from build123d import *

# Parameters (mm, degrees)
EXTRUDE_1_DEPTH = 3
EXTRUDE_START   = 3
SKETCH_2_R      = 1.35
SKETCH_2_R_2    = 3.25
EXTRUDE_2_DEPTH = 4
FILLET_1_R      = 5


with BuildPart() as part:
    # 草圖1 → 填料-伸長1 (new body)
    with BuildSketch(Plane.XY):
        with BuildLine():
            Line((25.7, -30), (25.7, 30))
            ThreePointArc((25.7, 30), (24.030508653, 34.030508653), (20, 35.7))
            Line((20, 35.7), (-20, 35.7))
            ThreePointArc((-20, 35.7), (-24.030508653, 34.030508653), (-25.7, 30))
            Line((-25.7, 30), (-25.7, -30))
            ThreePointArc((-25.7, -30), (-24.030508653, -34.030508653), (-20, -35.7))
            Line((-20, -35.7), (20, -35.7))
            ThreePointArc((20, -35.7), (24.030508653, -34.030508653), (25.7, -30))
        make_face()
    extrude(amount=EXTRUDE_1_DEPTH)

    # 草圖2 → 填料-伸長2 (add)
    with BuildSketch(Plane.XY.offset(EXTRUDE_START)):
        with BuildLine():
            Line((30, -30), (30, 30))
            ThreePointArc((30, 30), (27.071067812, 37.071067812), (20, 40))
            Line((20, 40), (-20, 40))
            ThreePointArc((-20, 40), (-27.071067812, 37.071067812), (-30, 30))
            Line((-30, 30), (-30, -30))
            ThreePointArc((-30, -30), (-27.071067812, -37.071067812), (-20, -40))
            Line((-20, -40), (20, -40))
            ThreePointArc((20, -40), (27.071067812, -37.071067812), (30, -30))
        make_face()
        with Locations((0, 38)):
            Circle(SKETCH_2_R, mode=Mode.SUBTRACT)
        with Locations((0, -38)):
            Circle(SKETCH_2_R, mode=Mode.SUBTRACT)
        Circle(SKETCH_2_R_2, mode=Mode.SUBTRACT)
        with Locations((14, 14)):
            Circle(SKETCH_2_R_2, mode=Mode.SUBTRACT)
    extrude(amount=EXTRUDE_2_DEPTH)

    # 圓角1
    # the kernel refuses this fillet: 5 mm, written as the material it takes off along each edge
    with BuildSketch(Plane(origin=(20, -30, 7), x_dir=(0, -1, 0), z_dir=(-1, 0, 0))) as fillet_1_piece_1:
        with BuildLine():
            CenterArc((5.101020514, -5), FILLET_1_R, 11.536959033, 78.463040967)
            Line((5.101020514, 0), (5.101020514, 0.1))
            Line((5.101020514, 0.1), (10, 0.1))
            Line((10, 0.1), (10.1, 0))
            ThreePointArc((10.1, 0), (10.1, -2), (10.09797959, -3.98))
            Line((10.09797959, -3.98), (10, -4))
        make_face()
    revolve(axis=Axis((20, -30, 7), (0, 0, 1)), revolution_arc=90, mode=Mode.SUBTRACT)
    with BuildSketch(Plane(origin=(30, -30, 7), x_dir=(-1.5640821970914211e-12, 0, -1.0), z_dir=(0, 1, 0)), Plane(origin=(-30, 30, 7), x_dir=(1.5640821970914211e-12, 0, -1.0), z_dir=(0, -1, 0))) as fillet_1_piece_2:
        with BuildLine():
            CenterArc((5, 4.898979486), FILLET_1_R, 180, 78.463040967)
            Line((0, 4.898979486), (-0.1, 4.898979486))
            Line((-0.1, 4.898979486), (-0.1, 0))
            Line((-0.1, 0), (0, -0.1))
            ThreePointArc((0, -0.1), (2, -0.1), (3.98, -0.09797959))
            Line((3.98, -0.09797959), (4, 0))
        make_face()
    extrude(amount=60, mode=Mode.SUBTRACT)
    with BuildSketch(Plane(origin=(20, 30, 7), x_dir=(1, 0, 0), z_dir=(0, -1, 0))) as fillet_1_piece_3:
        with BuildLine():
            CenterArc((5.101020514, -5), FILLET_1_R, 11.536959033, 78.463040967)
            Line((5.101020514, 0), (5.101020514, 0.1))
            Line((5.101020514, 0.1), (10, 0.1))
            Line((10, 0.1), (10.1, 0))
            ThreePointArc((10.1, 0), (10.1, -2), (10.09797959, -3.98))
            Line((10.09797959, -3.98), (10, -4))
        make_face()
    revolve(axis=Axis((20, 30, 7), (0, 0, 1)), revolution_arc=90, mode=Mode.SUBTRACT)
    with BuildSketch(Plane(origin=(20, 40, 7), x_dir=(0, -1.5667467323505197e-12, -1.0), z_dir=(-1, 0, 0)), Plane(origin=(-20, -40, 7), x_dir=(0, 1.5667467323505197e-12, -1.0), z_dir=(1, 0, 0))) as fillet_1_piece_4:
        with BuildLine():
            CenterArc((5, 4.898979486), FILLET_1_R, 180, 78.463040967)
            Line((0, 4.898979486), (-0.1, 4.898979486))
            Line((-0.1, 4.898979486), (-0.1, 0))
            Line((-0.1, 0), (0, -0.1))
            ThreePointArc((0, -0.1), (2, -0.1), (3.98, -0.09797959))
            Line((3.98, -0.09797959), (4, 0))
        make_face()
    extrude(amount=40, mode=Mode.SUBTRACT)
    with BuildSketch(Plane(origin=(-20, 30, 7), x_dir=(0, 1, 0), z_dir=(1, 0, 0))) as fillet_1_piece_5:
        with BuildLine():
            CenterArc((5.101020514, -5), FILLET_1_R, 11.536959033, 78.463040967)
            Line((5.101020514, 0), (5.101020514, 0.1))
            Line((5.101020514, 0.1), (10, 0.1))
            Line((10, 0.1), (10.1, 0))
            ThreePointArc((10.1, 0), (10.1, -2), (10.09797959, -3.98))
            Line((10.09797959, -3.98), (10, -4))
        make_face()
    revolve(axis=Axis((-20, 30, 7), (0, 0, 1)), revolution_arc=90, mode=Mode.SUBTRACT)
    with BuildSketch(Plane(origin=(-20, -30, 7), x_dir=(-1, 0, 0), z_dir=(0, 1, 0))) as fillet_1_piece_6:
        with BuildLine():
            CenterArc((5.101020514, -5), FILLET_1_R, 11.536959033, 78.463040967)
            Line((5.101020514, 0), (5.101020514, 0.1))
            Line((5.101020514, 0.1), (10, 0.1))
            Line((10, 0.1), (10.1, 0))
            ThreePointArc((10.1, 0), (10.1, -2), (10.09797959, -3.98))
            Line((10.09797959, -3.98), (10, -4))
        make_face()
    revolve(axis=Axis((-20, -30, 7), (0, 0, 1)), revolution_arc=90, mode=Mode.SUBTRACT)


solid = part.part
CAD build for the part. Positions are in the model's coordinates, mm. A direction names the side the tool comes from. Round coordinates to 2 decimals unless told otherwise and drop trailing zeros. Order: outer loops, then holes, each group sorted by start corner. A loop starts at its lowest first (then second) coordinate and runs counter-clockwise, first axis right, second up. Notation, with made-up numbers: M -31.75,14 L -3.75,14 A29 ccw -3.75,46 Z; hole C 20.5,5 d7. An arc over 180 degrees is marked long. Use one line per item in the form item = value.
Q1. Probe L1, parallel to Y at x = 0, z = 6; L2, parallel to Y at x = 0, z = 4.25; L3, parallel to Y at x = 17.5, z = 1.75. List the from-to ranges inside material, lowest first.
Recorded:
L1 = -36.65 to -3.25, 3.25 to 36.65
L2 = -39.57 to -39.35, -36.65 to -3.25, 3.25 to 36.65, 39.35 to 39.57
L3 = -35.7 to 35.7
Q2. Saw through at D-D on y = 22.5. Give the cut face in (x, z), then the cut area to 3 significant figures.
Recorded:
outline = M -30,3 L -25.7,3 L -25.7,0 L 25.7,0 L 25.7,3 L 30,3 A5 ccw 25.1,7 L -25.1,7 A5 ccw Z
area = 384 mm^2
Q3. Which spindle directions (+Z, -Z, +X, -X, +Y, -Y) get a long thin tool onto all of the face, cutting with end or side? Do faces 1 (the flat face through (-27, 6, 3)), 2 (the flat face through (-25.7, 0, 1)), 3 (the cylindrical face through (24.07, 33.99, 1.48)). Say none if no direction does.
Recorded:
face_1 = -Z
face_2 = -Z, -X, +Y, -Y
face_3 = -Z, +X, +Y
Q4. Two-plate mould, pull along X, no slides. Class faces 4 (the cylindrical face through (23.99, -34.07, 1.48)), 5 (the cylindrical face through (10.753, 14.143, 4.972)), 6 (the flat face through (-6, 0, 7)): +X half, -X half, draft (parallel to the pull), parting line (faces both ways), or undercut.
Recorded:
face_4 = +X half
face_5 = undercut
face_6 = draft
Q5. Saw through at A-A on y = 14. Give the cut face in (x, z), then the cut area to 3 significant figures.
Recorded:
outline = M -30,3 L -25.7,3 L -25.7,0 L 25.7,0 L 25.7,3 L 30,3 A5 ccw 25.1,7 L 17.25,7 L 17.25,3 L 10.75,3 L 10.75,7 L -25.1,7 A5 ccw Z
area = 358 mm^2
Q6. Saw through at B-B on x = 0. Give the cut face in (y, z), then the cut area to 3 significant figures.
Recorded:
outline = M -40,3 L -39.35,3 L -39.35,4.64 A5 ccw Z; M -36.65,3 L -35.7,3 L -35.7,0 L 35.7,0 L 35.7,3 L 36.65,3 L 36.65,6.75 A5 ccw 35.1,7 L 3.25,7 L 3.25,3 L -3.25,3 L -3.25,7 L -35.1,7 A5 ccw -36.65,6.75 Z; M 39.35,3 L 40,3 A5 ccw 39.35,4.64 Z
area = 482 mm^2
Q7. Flat gauge pins, fed straight in: P1, Ø2.5, axis at y = -7, z = 1.5, coming from the -X side; P2, Ø6, axis at x = 0, y = 0, coming from the -Z side; P3, Ø3, axis at x = 0, y = -38, coming from the +Z side; P4, Ø1, axis at y = -3.5, z = 4, coming from the +X side. Where does each tip first touch, or does it go through?
Recorded:
P1 = -25.7
P2 = 0
P3 = 6.8
P4 = 29.87
Q8. Saw through at C-C on z = 2. Give the cut face in (x, y), then the cut area to 3 significant figures.
Recorded:
outline = M -25.7,-30 A5.7 ccw -20,-35.7 L 20,-35.7 A5.7 ccw 25.7,-30 L 25.7,30 A5.7 ccw 20,35.7 L -20,35.7 A5.7 ccw -25.7,30 Z
area = 3,640 mm^2
